The model under review builds one solid part; all positions refer to its coordinate system, in mm. Face numbers are marked on the shaded views. A direction names the side the tool comes from. Round coordinates to 2 decimals unless told otherwise and drop trailing zeros. Loops run counter-clockwise (first coordinate to the right, second up) from the corner with the lowest first, then second, coordinate; pieces in that order, holes last. Notation, with made-up numbers: (19.5, 2) -> (42.5, 2) arc R19 ccw to (42.5, 16) -> close; hole circle Ø7 at (41, 24). An arc over 180 degrees is marked (long way). Write each question's results on one line, items separated by ' | '. Start each with the question number.
Item 1: We need section A-A (y = 16). Give the boundary of the cut face in (x, z), and give its area (3 significant figures).
Item 2: Tool access review of the marked faces 4 and 5: name each direction out of +Z, -Z, +X, -X, +Y, -Y from which nothing blocks a thin tool from reaching the whole face with its end or side.
Item 3: We need section C-C (x = 8.75). Give the boundary of the cut face in (y, z), and give its area (3 significant figures).
Item 4: We need section B-B (x = 0). Give the boundary of the cut face in (y, z) (3 decimals), and give its area (3 significant figures).
Item 5: Mouldability with a two-part tool opening along Y and no side actions: class the marked faces 1, 2 and 3 as pulls with the +Y half, pulls with the -Y half, needs draft (parallel to the pull), parting line crosses it, or undercut.
Item 6: Clearance check with flat-ended pins moving along their axes: pin 1 Ø6 at (x, y) = (-3.5, 58.5) entering from +Z; pin 2 Ø14 at (y, z) = (17, 23) entering from -X; pin 3 Ø12 at (x, y) = (-1.5, 17.5) entering from +Z; pin 4 Ø2 at (x, z) = (-4.5, 51) entering from -Y. State where each tip first meets the part, or that it passes through.
Item 7: We need section D-D (y = 46.5). Give the boundary of the cut face in (x, z).
Item 8: For L1, parallel to X at y = 11, z = 8; L2, parallel to Z at x = 7, y = 51.5; L3, parallel to Z at x = 3.75, y = 20.5, list the stretches that pass through material, from the lowest coordinate up. Write a range as from..to.
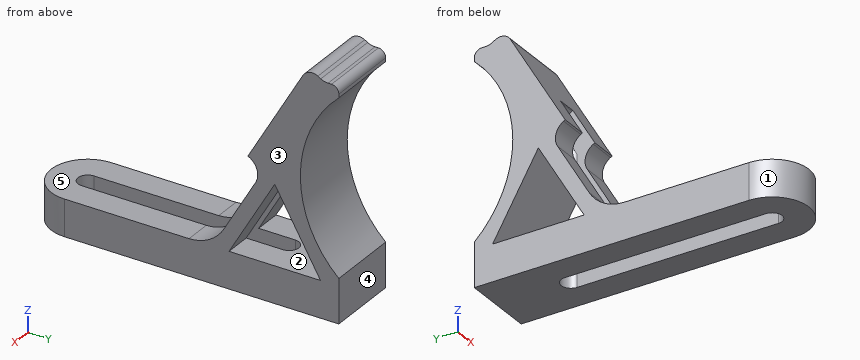
from build123d import *

# Parameters (mm, degrees)
PAD_DEPTH       = 67.31
POCKET_DEPTH    = 20.001
POCKET001_DEPTH = 62.936332
FILLET_R        = 11
PAD001_DEPTH    = 5
FILLET001_R     = 4.5
FILLET002_R     = 4.75
FILLET003_R     = 3
FILLET004_R     = 4
FILLET005_R     = 2


with BuildPart() as part:
    # Sketch → Pad (new body)
    with BuildSketch(Plane.XY):
        with BuildLine():
            Line((-10, 75), (-10, 0))
            ThreePointArc((-10, 0), (0, -10), (10, 0))
            Line((10, 0), (10, 75))
            Line((10, 75), (-10, 75))
        make_face()
    extrude(amount=PAD_DEPTH)

    # Sketch001 (on Face1 of Pad) → Pocket (cut, through all)
    with BuildSketch(Plane(origin=(-10, 0, 0), x_dir=(0, -1, 0), z_dir=(-1, 0, 0))):
        Polygon((-71, 62.935332), (-40.437772, 10), (26.946924, 10), (26.946924, 74.479118), (-81.836647, 74.479118), (-81.836647, 62.935332), align=None)
        with BuildLine():
            ThreePointArc((-75, 12.064668), (-64.49, 36), (-75, 59.935332))
            Line((-75, 59.935332), (-97, 36))
            Line((-97, 36), (-75, 12.064668))
        make_face()
        Polygon((-70, 10), (-45, 10), (-57.5, 31.650635), align=None)
    extrude(amount=-POCKET_DEPTH, mode=Mode.SUBTRACT)

    # Sketch002 (on Face2 of Pocket) → Pocket001 (cut, through all)
    with BuildSketch(Plane(origin=(0, 0, 0), x_dir=(1, 0, 0), z_dir=(0, 0, -1))):
        with BuildLine():
            ThreePointArc((2.667, 0), (0, 2.667), (-2.667, 0))
            Line((-2.667, 0), (-2.667, -55))
            ThreePointArc((-2.667, -55), (0, -57.667), (2.667, -55))
            Line((2.667, 0), (2.667, -55))
        make_face()
    extrude(amount=-POCKET001_DEPTH, mode=Mode.SUBTRACT)

    # Fillet
    fillet_edges = [part.edges().sort_by_distance(p)[0] for p in [
        (6.3335, 40.437772, 10),
        (-6.3335, 40.437772, 10),
    ]]
    fillet(fillet_edges, radius=FILLET_R)

    # Sketch003 (on Face5 of Fillet) → Pad001 (join)
    with BuildSketch(Plane(origin=(0, 25.998202, -15.010069), x_dir=(1, 0, 0), z_dir=(0, -0.866025, 0.5))):
        Polygon((-10, 90.003596), (10, 90.003596), (10, 57.003596), (2.667, 57.003596), (2.667, 69.003596), (-2.667, 69.003596), (-2.667, 57.003596), (-10, 57.003596), align=None)
    extrude(amount=PAD001_DEPTH)

    # Fillet001
    fillet001_edges = [part.edges().sort_by_distance(p)[0] for p in [
        (6.3335, 54.5, 34.356493),
        (-6.3335, 54.5, 34.356493),
    ]]
    fillet(fillet001_edges, radius=FILLET001_R)

    # Fillet002
    fillet002_edges = [part.edges().sort_by_distance(p)[0] for p in [
        (0, 60.5, 44.748798),
    ]]
    fillet(fillet002_edges, radius=FILLET002_R)

    # Fillet003
    fillet003_edges = [part.edges().sort_by_distance(p)[0] for p in [
        (0, 66.669873, 65.435332),
    ]]
    fillet(fillet003_edges, radius=FILLET003_R)

    # Fillet004
    fillet004_edges = [part.edges().sort_by_distance(p)[0] for p in [
        (0, 71, 62.935332),
    ]]
    fillet(fillet004_edges, radius=FILLET004_R)

    # Fillet005
    fillet005_edges = [part.edges().sort_by_distance(p)[0] for p in [
        (0, 75, 62.935332),
    ]]
    fillet(fillet005_edges, radius=FILLET005_R)


solid = part.part
Here are the results:
1) outline: (-10, 0) -> (-2.67, 0) -> (-2.67, 10) -> (-10, 10) -> close; (2.67, 0) -> (10, 0) -> (10, 10) -> (2.67, 10) -> close | area: 147 mm2
2) face 4: +Z, -Z, +X, -X, +Y | face 5: +Z, +X, -X, -Y
3) outline: (-4.84, 0) -> (75, 0) -> (75, 12.06) arc R32.51 cw to (75, 59.94) -> (75, 60.94) arc R2 ccw to (73, 62.94) -> (72.07, 62.94) arc R4 cw to (70.07, 63.47) -> (69.27, 63.94) arc R3 ccw to (65.17, 62.84) -> (50.17, 36.86) -> (50.6, 36.61) arc R4.5 cw to (52.25, 30.46) -> (43.61, 15.5) arc R11 cw to (34.09, 10) -> (-4.84, 10) -> close; hole (45, 10) -> (70, 10) -> (57.5, 31.65) -> close | area: 1,370 mm2
4) outline: (-10, 0) -> (-2.667, 0) -> (-2.667, 10) -> (-10, 10) -> close; (56.17, 47.249) -> (56.386, 47.124) arc R4.75 cw to (58.125, 40.635) -> (57.667, 39.842) -> (57.667, 31.361) -> (70, 10) -> (57.667, 10) -> (57.667, 0) -> (75, 0) -> (75, 12.065) arc R32.51 cw to (75, 59.935) -> (75, 60.935) arc R2 ccw to (73, 62.935) -> (72.072, 62.935) arc R4 cw to (70.072, 63.471) -> (69.268, 63.935) arc R3 ccw to (65.17, 62.837) -> close | area: 638 mm2
5) face 1: pulls with the -Y half | face 2: undercut | face 3: needs draft
6) pin 1: stops at z = 56.48 | pin 2: passes through | pin 3: stops at z = 10 | pin 4: stops at y = 57.76
7) outline: (-10, 0) -> (-2.67, 0) -> (-2.67, 10) -> (-10, 10) -> close; (-10, 12.6) -> (-2.67, 12.6) -> (-2.67, 20.5) -> (-10, 20.5) -> close; (2.67, 0) -> (10, 0) -> (10, 10) -> (2.67, 10) -> close; (2.67, 12.6) -> (10, 12.6) -> (10, 20.5) -> (2.67, 20.5) -> close
8) L1: x = -10..-2.67, 2.67..10 | L2: z = 0..10, 21.26..29.16, 35.93..39.16 | L3: z = 0..10
